Can you work these out from the model? Positions are in its coordinate system, mm. A direction names the side the tool comes from. Coordinates: 2 decimals unless noted, no trailing zeros. Write each loop counter-clockwise with the first axis right and the second up, starting at its lowest first coordinate (ties: lowest second). Pieces come first, ordered by that corner, then holes.
```python
from build123d import *

# Parameters (mm, degrees)
SKETCH049_W      = 1
SKETCH049_H      = 1
EXTRUDE052_DEPTH = 8.5
SKETCH048_W      = 2.4
SKETCH048_H      = 2.4
EXTRUDE051_DEPTH = 8.5
SKETCH046_W      = 5.2
SKETCH046_H      = 5.2
EXTRUDE049_DEPTH = 1
SKETCH047_W      = 10
SKETCH047_H      = 10.2
EXTRUDE050_DEPTH = 8
SKETCH045_W      = 7
SKETCH045_H      = 10.2
EXTRUDE048_DEPTH = 8.5


with BuildPart() as extrude052:
    # Sketch049 → Extrude052 (new body, symmetric)
    with BuildSketch(Plane.XZ):
        with Locations((1.5, -4.6)):
            Rectangle(SKETCH049_W, SKETCH049_H)
        with Locations((1.5, 4.6)):
            Rectangle(SKETCH049_W, SKETCH049_H)
    extrude(amount=EXTRUDE052_DEPTH, both=True)


with BuildPart() as obj1:
    # Sketch048 → Extrude051 (new body, symmetric)
    with BuildSketch(Plane.XZ):
        with Locations((4.2, 0)):
            Rectangle(SKETCH048_W, SKETCH048_H)
    extrude(amount=EXTRUDE051_DEPTH, both=True)


with BuildPart() as obj2:
    # Sketch046 → Extrude049 (new body)
    with BuildSketch(Plane.YZ):
        Rectangle(SKETCH046_W, SKETCH046_H)
    extrude(amount=EXTRUDE049_DEPTH)


with BuildPart() as obj3:
    # Sketch047 → Extrude050 (new body)
    with BuildSketch(Plane.YZ):
        Rectangle(SKETCH047_W, SKETCH047_H)
    extrude(amount=EXTRUDE050_DEPTH)


with BuildPart() as obj3_1:
    # Extrude050 placement: moved
    add(obj3.part.moved(Location((1, 0, 0))))


with BuildPart() as obj4:
    # Sketch045 → Extrude048 (new body, symmetric)
    with BuildSketch(Plane.XZ):
        with Locations((3.5, 0)):
            Rectangle(SKETCH045_W, SKETCH045_H)
    extrude(amount=EXTRUDE048_DEPTH, both=True)

    # Cut030: cut obj3
    add(obj3_1.part, mode=Mode.SUBTRACT)

    # Cut031: cut obj2
    add(obj2.part, mode=Mode.SUBTRACT)

    # Cut032: cut obj1
    add(obj1.part, mode=Mode.SUBTRACT)

    # Fusion001: union Extrude052
    add(extrude052.part)


solid = obj4.part
```
1. We'd pull the mould along Y, two halves only. Please class faces 1 (the face through (2.7, 8.5, 0.1)), 2 (the face through (0.5, 0, -2.6)), 3 (the face through (4, 7, 1.2)): released by +Y, released by -Y, zero draft, split by the parting line, or undercut.
2. Which directions (+Z, -Z, +X, -X, +Y, -Y) give clear straight access to the entire face, cutting with the end or side of a thin tool? Please do faces 4 (the face through (4, -7, 1.2)), 5 (the face through (7, 7, 0)), 6 (the face through (2, 0.1, -4.6)), 7 (the face through (0.5, 2.6, 0)), 8 (the face through (1.5, 0.1, -4.1)).
3. If we section it at C-C, the plane y = 2: List the corners of the cut face in (x, z) for me.
4. If we section it at B-B, the plane z = -1: List the corners of the cut face in (x, y) for me.
5. If we section it at D-D, the plane x = 0.5: List the corners of the cut face in (y, z) for me.
6. I'm going to push a flat-ended pin straight in: P1, Ø1.5, axis at y = -4, z = -0.5, coming from the +X side. Where does the tip first touch, or does it pass through?
7. If I drill on L1, parallel to Y at x = 4.75, z = 2; L2, parallel to Z at x = 1.5, y = 2.25; L3, parallel to Z at x = 5.25, y = 7, over which ranges is the centre line in solid material (lowest first)?
8. If we section it at A-A, the plane x = 4.5: List the corners of the cut face in (y, z) for me.
Answers:
1. face 1: released by +Y
1. face 2: undercut
1. face 3: zero draft
2. face 4: +Y, -Y
2. face 5: +Z, -Z, +X, +Y, -Y
2. face 6: +Z, -Z, +X
2. face 7: +X, -X
2. face 8: +X
3. outline: (0, -5.1) - (2, -5.1) - (2, -4.1) - (1, -4.1) - (1, -2.6) - (0, -2.6) - close; (0, 2.6) - (1, 2.6) - (1, 4.1) - (2, 4.1) - (2, 5.1) - (0, 5.1) - close
4. outline: (0, -8.5) - (3, -8.5) - (3, -5) - (1, -5) - (1, -2.6) - (0, -2.6) - close; (0, 2.6) - (1, 2.6) - (1, 5) - (3, 5) - (3, 8.5) - (0, 8.5) - close; (5.4, -8.5) - (7, -8.5) - (7, -5) - (5.4, -5) - close; (5.4, 5) - (7, 5) - (7, 8.5) - (5.4, 8.5) - close
5. outline: (-8.5, -5.1) - (8.5, -5.1) - (8.5, 5.1) - (-8.5, 5.1) - close; hole (-2.6, -2.6) - (2.6, -2.6) - (2.6, 2.6) - (-2.6, 2.6) - close
6. P1: stops at x = 1
7. L1: y = -8.5 to -5, 5 to 8.5
7. L2: z = -5.1 to -4.1, 4.1 to 5.1
7. L3: z = -5.1 to -1.2, 1.2 to 5.1
8. outline: (-8.5, -5.1) - (-5, -5.1) - (-5, -1.2) - (-8.5, -1.2) - close; (-8.5, 1.2) - (-5, 1.2) - (-5, 5.1) - (-8.5, 5.1) - close; (5, -5.1) - (8.5, -5.1) - (8.5, -1.2) - (5, -1.2) - close; (5, 1.2) - (8.5, 1.2) - (8.5, 5.1) - (5, 5.1) - close
